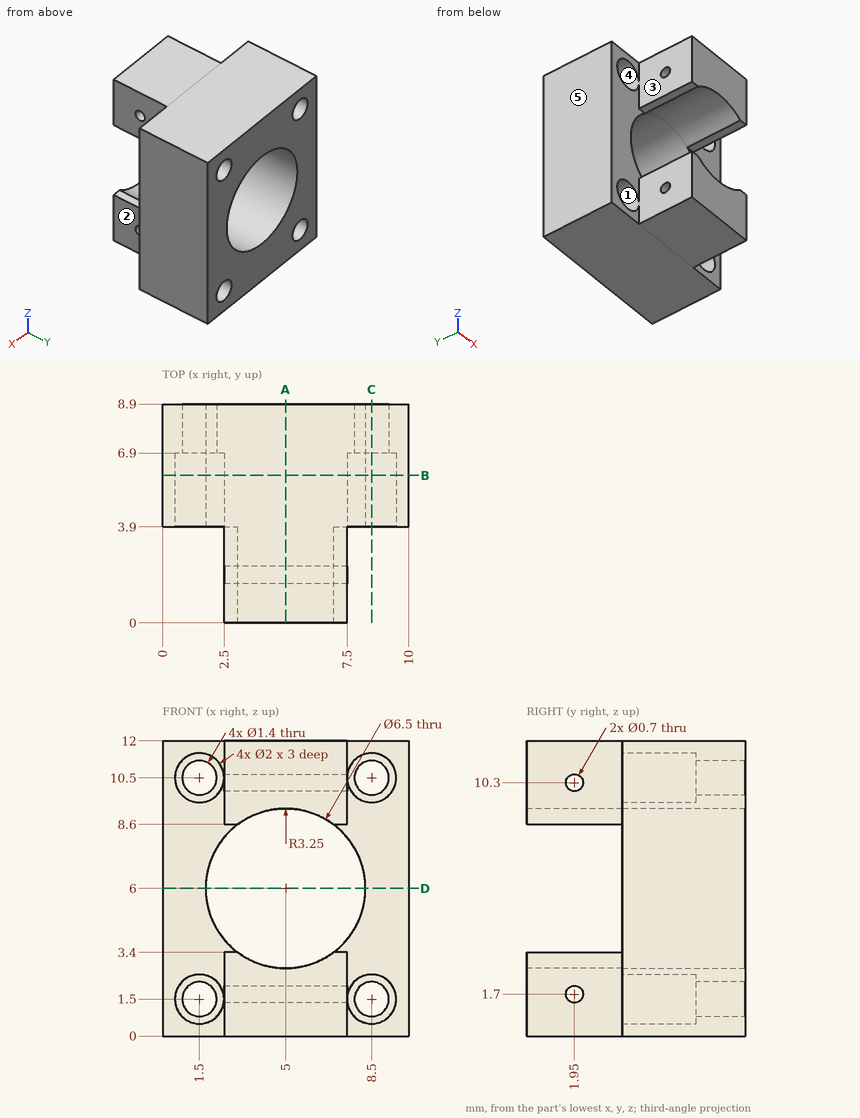
Check sheet for the drawn part. Datum: minimum x, y, z corner. Units: mm. A direction names the side the tool comes from. Give positions to 0.01 mm unless a question says otherwise; leave off trailing zeros. Write each loop counter-clockwise with the first axis right and the second up, starting at its lowest first coordinate (ties: lowest second). Pieces come first, ordered by that corner, then holes. Notation, with made-up numbers: (-9.5, -6) - (22.5, -6) arc R23 cw to (22.5, 20) - close; hole circle Ø8 at (6, -7.5). An arc over 180 degrees is marked (long way). Put each result on its own line as item: value.
1. Sectioned sample at D-D, the plane z = 6. Enter the section's corners in (x, y).
Ans:
outline: (0, 3.9) - (1.75, 3.9) - (1.75, 8.9) - (0, 8.9) - close; (8.25, 3.9) - (10, 3.9) - (10, 8.9) - (8.25, 8.9) - close
2. Set-up check for the marked faces 1, 2 and 3: record each of +Z, -Z, +X, -X, +Y, -Y from which the full face is reachable in a straight line by a thin tool's end or side.
Ans:
face 1: -Y
face 2: +Z, -Z, +X, -Y
face 3: +Z, -Z, -X, -Y
3. Thickness scan on line 1 (X direction, y = 7.4, z = 10.5); line 2 (Y direction, x = 4.15, z = 1.7); line 3 (X direction, y = 5.1, z = 1.5). Record the ranges inside material, lowest first.
Ans:
line 1: x = 0 to 0.8, 2.2 to 7.8, 9.2 to 10
line 2: y = 0 to 1.6, 2.3 to 8.9
line 3: x = 0 to 0.5, 2.5 to 7.5, 9.5 to 10
4. Go/stop test with flat-tipped pins: pin 1 (0.9 mm diameter, centred on x = 2, z = 5, fed in from -Y); pin 2 (1 mm diameter, centred on y = 2.5, z = 11, fed in from -X); pin 3 (1 mm diameter, centred on y = 2.5, z = 10.5, fed in from +X). Record where each tip stops, or that it passes through.
Ans:
pin 1: stops at y = 3.9
pin 2: stops at x = 2.5
pin 3: stops at x = 7.5
5. Sectioned sample at B-B, the plane y = 6. Enter the section's corners in (x, z).
Ans:
outline: (0, 0) - (10, 0) - (10, 12) - (0, 12) - close; hole circle Ø2 at (1.5, 1.5); hole circle Ø2 at (1.5, 10.5); hole circle Ø6.5 at (5, 6); hole circle Ø2 at (8.5, 1.5); hole circle Ø2 at (8.5, 10.5)
6. Sectioned sample at A-A, the plane x = 5. Enter the section's corners in (y, z).
Ans:
outline: (0, 0) - (8.9, 0) - (8.9, 2.75) - (0, 2.75) - close; (0, 9.25) - (8.9, 9.25) - (8.9, 12) - (0, 12) - close; hole circle Ø0.7 at (1.95, 1.7); hole circle Ø0.7 at (1.95, 10.3)
7. Draft check along Z on the marked faces 4 and 5. Enter one of: +Z half, -Z half, draft (parallel to the pull), parting line (faces both ways), or undercut.
Ans:
face 4: undercut
face 5: draft
8. Sectioned sample at C-C, the plane x = 8.5. Enter the section's corners in (y, z), plus the area to 3 significant figures.
Ans:
outline: (3.9, 0) - (8.9, 0) - (8.9, 0.8) - (6.9, 0.8) - (6.9, 0.5) - (3.9, 0.5) - close; (3.9, 2.5) - (6.9, 2.5) - (6.9, 2.2) - (8.9, 2.2) - (8.9, 9.8) - (6.9, 9.8) - (6.9, 9.5) - (3.9, 9.5) - close; (3.9, 11.5) - (6.9, 11.5) - (6.9, 11.2) - (8.9, 11.2) - (8.9, 12) - (3.9, 12) - close
area: 42.4 mm²
